from build123d import *

# Parameters (mm, degrees)
F0_R     = 10.0661107962
F1_DEPTH = 381


with BuildPart() as f1:
    # F0 (on Front) → F1 (new body)
    with BuildSketch(Plane.XZ):
        with BuildLine():
            ThreePointArc((-460.4171146545, -80.3520751223), (-528.7422428891, -234.5899299241), (-545.0866186853, -402.490199078))
            Line((-545.0866186853, -402.490199078), (-306.3518632039, -402.490199078))
            ThreePointArc((-306.3518632039, -402.490199078), (-211.6500630521, -231.3956211083), (-61.0918521756, -356.1914972432))
            ThreePointArc((-61.0918521756, -356.1914972432), (-63.2959760406, -379.7497081198), (-69.8318411473, -402.490199078))
            Line((-69.8318411473, -402.490199078), (281.923010605, -402.490199078))
            ThreePointArc((281.923010605, -402.490199078), (369.5574089397, -199.0626294837), (544.651634751, -334.7260951996))
            ThreePointArc((544.651634751, -334.7260951996), (540.2117829098, -369.7170034539), (527.173623783, -402.490199078))
            Line((527.173623783, -402.490199078), (587.5886353005, -402.490199078))
            ThreePointArc((587.5886353005, -402.490199078), (614.2875363688, -399.5230484268), (640.7299934295, -394.7868299108))
            ThreePointArc((640.7299934295, -394.7868299108), (656.2355333133, -185.0675662335), (556.3726911105, 0))
            Line((556.3726911105, 0), (-226.5663393053, -61.8719576371))
            Line((-226.5663393053, -61.8719576371), (-409.496628924, -76.3280706806))
            Line((-409.496628924, -76.3280706806), (-460.4171146545, -80.3520751223))
        make_face()
        with BuildLine():
            ThreePointArc((0, 185.9708741245), (-127.8124548077, 75.3314520254), (-226.5663393053, -61.8719576371))
            Line((-226.5663393053, -61.8719576371), (556.3726911105, 0))
            ThreePointArc((556.3726911105, 0), (558.7501920915, 120.3142873349), (510.4560028632, 230.5361160923))
            ThreePointArc((510.4560028632, 230.5361160923), (254.2993354525, 218.8905544569), (0, 185.9708741245))
        make_face()
        with BuildLine():
            ThreePointArc((-61.0918521756, -356.1914972432), (-211.6500630521, -231.3956211083), (-306.3518632039, -402.490199078))
            Line((-306.3518632039, -402.490199078), (-69.8318411473, -402.490199078))
            ThreePointArc((-69.8318411473, -402.490199078), (-63.2959760406, -379.7497081198), (-61.0918521756, -356.1914972432))
        make_face()
        with Locations((-188.0918521756, -356.1914972432)):
            Circle(F0_R, mode=Mode.SUBTRACT)
        with BuildLine():
            Line((-69.8318411473, -402.490199078), (-306.3518632039, -402.490199078))
            ThreePointArc((-306.3518632039, -402.490199078), (-188.0918521756, -483.1914972432), (-69.8318411473, -402.490199078))
        make_face()
        with BuildLine():
            ThreePointArc((544.651634751, -334.7260951996), (369.5574089397, -199.0626294837), (281.923010605, -402.490199078))
            Line((281.923010605, -402.490199078), (527.173623783, -402.490199078))
            ThreePointArc((527.173623783, -402.490199078), (540.2117829098, -369.7170034539), (544.651634751, -334.7260951996))
        make_face()
        with BuildLine():
            Line((527.173623783, -402.490199078), (281.923010605, -402.490199078))
            ThreePointArc((281.923010605, -402.490199078), (404.548317194, -474.8294127566), (527.173623783, -402.490199078))
        make_face()
    extrude(amount=F1_DEPTH)


solid = f1.part
Here's how the part is built. I have some questions about the finished solid (model axes, mm). A direction names the side the tool comes from. Coordinates: 2 decimals unless noted, no trailing zeros. Order: outer loops, then holes, each group sorted by start corner. A loop starts at its lowest first (then second) coordinate and runs counter-clockwise, first axis right, second up. Notation, with made-up numbers: M 86.25,-11.5 L 106.25,-11.5 A8 ccw 106.25,-5.5 Z; hole C 72.5,-36.5 d3. An arc over 180 degrees is marked long. Answer as CSV lines item,"result". Start each with the question number.
1. We'd pull the mould along Z, two halves only. Please class faces 1 (the cylindrical face through (613.915, -187.833, -399.577)), 2 (the flat face through (185, -381, -121)), 3 (the cylindrical face through (257.88, -187.83, 219.2)), 4 (the cylindrical face through (559.077, -187.833, 118.648)): released by +Z, released by -Z, zero draft, split by the parting line, or undercut.
2. I want a section at C-C, the plane x = 100. Write out the boundary of the cut face in (y, z), and give its area (3 significant figures).
3. I want a section at B-B, the plane z = 131.5. Write out the boundary of the cut face in (x, y), and give its area (3 significant figures).
4. I want a section at A-A, the plane y = -203. Write out the boundary of the cut face in (x, z), and give its area (3 significant figures).
5. On a 3-axis mill with a long thin cutter (end or side, diameter ignored), from which of +Z, -Z, +X, -X, +Y, -Y can I reach the whole of each face in a straight line? I mean faces 5 (the flat face through (557, -188, -402.49)), 6 (the flat face through (185, 0, -121)), 7 (the flat face through (-427, -188, -402.49)), 8 (the flat face through (-341.855, -187.833, -70.983)), 9 (the flat face through (104, -188, -402.49)). Say none if no direction works.
6. I need wall thicknesses on line 1 (Z direction, x = 438, y = -113); line 2 (Z direction, x = 258, y = -81.5); line 3 (X direction, y = -306.5, z = 106). Which ranges of each line are inside material? Lowest first, please. Write a range as [from, to].
7. For pin 1 (1 mm diameter, centred on x = 217, y = -223, fed in from -Z); pin 2 (12 mm diameter, centred on y = -105.5, z = -176.5, fed in from +X); pin 3 (3 mm diameter, centred on y = -245, z = 84.5, fed in from -X), each with a flat end and sliding along its axis, tell me the tip position at first contact or that it passes through.
Recorded:
1,face 1,"released by -Z"
1,face 2,"zero draft"
1,face 3,"released by +Z"
1,face 4,"undercut"
2,outline,"M -381,-402.49 L 0,-402.49 L 0,201.49 L -381,201.49 Z"
2,area,"230,000 mm2"
3,outline,"M -70.45,-381 L 556.28,-381 L 556.28,0 L -70.45,0 Z"
3,area,"239,000 mm2"
4,outline,"M -545.09,-402.49 L -306.35,-402.49 A127 ccw -69.83,-402.49 L 281.92,-402.49 A140.1 ccw 527.17,-402.49 L 587.59,-402.49 A403.7 ccw 640.73,-394.79 A374.85 ccw 556.37,0 A280.28 ccw 510.46,230.54 A3078.99 ccw 0,185.97 A725.85 ccw -226.57,-61.87 L -460.42,-80.35 A529.48 ccw Z; hole C -188.09,-356.19 d20.13"
4,area,"609,000 mm2"
5,face 5,"-Z, +X, +Y, -Y"
5,face 6,"+Z, -Z, +X, -X, +Y"
5,face 7,"-Z, -X, +Y, -Y"
5,face 8,"+Z, -X, +Y, -Y"
5,face 9,"-Z, +Y, -Y"
6,line 1,"z = [-470.78, 229.41]"
6,line 2,"z = [-402.49, 219.21]"
6,line 3,"x = [-98.07, 561.22]"
7,pin 1,"stops at z = -402.49"
7,pin 2,"stops at x = 655.68"
7,pin 3,"stops at x = -120.7"
